from build123d import *

# Parameters (mm, degrees)
F1_DEPTH = 1548.47
F2_R     = 14
F3_DEPTH = 5
F4_R     = 9.5
F5_DEPTH = 5


with BuildPart() as f1:
    # F0 (on Right) → F1 (new body)
    with BuildSketch(Plane.YZ):
        Polygon((0, 0), (0, 100), (-5, 100), (-5, 5), (-100, 5), (-100, 0), align=None)
    extrude(amount=F1_DEPTH)

    # F2 (on face) → F3 (cut, through all)
    with BuildSketch(Plane.XY.offset(5)):
        with Locations((474.22, -52.5)):
            Circle(F2_R)
        with Locations((1074.22, -52.5)):
            Circle(F2_R)
        with Locations((1460.47, -52.5)):
            Circle(F2_R)
        with Locations((88, -52.5)):
            Circle(F2_R)
    extrude(amount=-F3_DEPTH, mode=Mode.SUBTRACT)

    # F4 (on Front) → F5 (cut, through all)
    with BuildSketch(Plane.XZ):
        with Locations((1267.47, 52.5)):
            Circle(F4_R)
        with Locations((881.22, 52.5)):
            Circle(F4_R)
        with Locations((544.22, 52.5)):
            Circle(F4_R)
        with Locations((281, 52.5)):
            Circle(F4_R)
    extrude(amount=F5_DEPTH, mode=Mode.SUBTRACT)


solid = f1.part
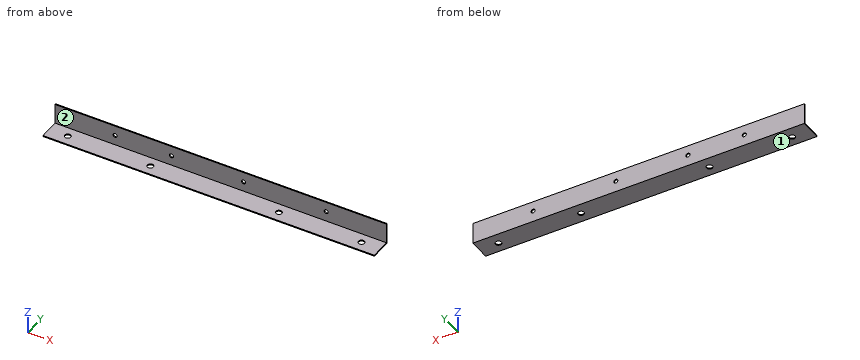
CAD build for the part. Positions are in the model's coordinates, mm. Face numbers are marked on the shaded views. A direction names the side the tool comes from. Round coordinates to 2 decimals unless told otherwise and drop trailing zeros. Write each loop counter-clockwise with the first axis right and the second up, starting at its lowest first coordinate (ties: lowest second). Pieces come first, ordered by that corner, then holes. Notation, with made-up numbers: M -3,24.25 L 29,24.25 A22 cw 29,36.25 Z; hole C -24.5,-33 d4. An arc over 180 degrees is marked long. Use a Markdown table: item, result. Add a question column.
1. Slice it at A-A on y = -52.5. Give the cut face in (x, z), then the cut area to 3 significant figures.
2. Flat gauge pins, fed straight in: P1, Ø3, axis at x = 797, y = -69.5, coming from the +Z side; P2, Ø8, axis at x = 539.5, z = 31, coming from the +Y side; P3, Ø25, axis at x = 1074.22, y = -52.5, coming from the -Z side; P4, Ø24.5, axis at x = 281, z = 52.5, coming from the -Y side. Where does each tip first touch, or does it go through?
3. Slice it at C-C on x = 320.5. Give the cut face in (y, z).
4. Slice it at D-D on z = 22.5. Give the cut face in (x, y).
5. Drill centre lines: probe 1 along Z at (x, y) = (281, -2); probe 2 along Z at (x, y) = (322, -79); probe 3 along Y at (x, z) = (754.5, 22). Where is each one in solid material? Low to high.
6. Slice it at B-B on x = 1460.47. Give the cut face in (y, z).
7. 3-axis set-ups, long thin cutter, end or side, ignore diameter. For the marked faces 1 and 2: which of +Z, -Z, +X, -X, +Y, -Y reach the whole face in a straight line?
Reply:
| question | item | result |
|---|---|---|
| 1 | outline | M 0,0 L 74,0 L 74,5 L 0,5 Z; M 102,0 L 460.22,0 L 460.22,5 L 102,5 Z; M 488.22,0 L 1060.22,0 L 1060.22,5 L 488.22,5 Z; M 1088.22,0 L 1446.47,0 L 1446.47,5 L 1088.22,5 Z; M 1474.47,0 L 1548.47,0 L 1548.47,5 L 1474.47,5 Z |
| 1 | area | 7,180 mm^2 |
| 2 | P1 | stops at z = 5 |
| 2 | P2 | stops at y = 0 |
| 2 | P3 | passes through |
| 2 | P4 | stops at y = -5 |
| 3 | outline | M -100,0 L 0,0 L 0,100 L -5,100 L -5,5 L -100,5 Z |
| 4 | outline | M 0,-5 L 1548.47,-5 L 1548.47,0 L 0,0 Z |
| 5 | probe 1 | z = 0 to 43, 62 to 100 |
| 5 | probe 2 | z = 0 to 5 |
| 5 | probe 3 | y = -5 to 0 |
| 6 | outline | M -100,0 L -66.5,0 L -66.5,5 L -100,5 Z; M -38.5,0 L 0,0 L 0,100 L -5,100 L -5,5 L -38.5,5 Z |
| 7 | face 1 | -Z, +X, -X, +Y, -Y |
| 7 | face 2 | +Z, +X, -X, -Y |
